The listing builds one solid part. Answer for the finished solid, in the listing's coordinates (mm). A direction names the side the tool comes from. Coordinates: 2 decimals unless noted, no trailing zeros. Loops run counter-clockwise (first coordinate to the right, second up) from the corner with the lowest first, then second, coordinate; pieces in that order, holes last. Notation, with made-up numbers: (68, -23) -> (84, -23) arc R28 ccw to (84, -5) -> close; hole circle Ø2 at (55.5, 70.5). An arc over 180 degrees is marked (long way). Answer in a Markdown table with one row per item.
```python
from build123d import *

# Parameters (mm, degrees)
SKETCH_1_R                   = 14
EXTRUDE_1_DEPTH              = 6
HOLE_WIZARD_M4_3_D           = 4.5
HOLE_WIZARD_M4_3_CBORE_D     = 8
HOLE_WIZARD_M4_3_CBORE_DEPTH = 4.4
PATTERN_CIRCULAR_1_COUNT     = 4
CHAMFER_1_SIZE               = 0.2


with BuildPart() as part:
    # 草圖1 → 填料-伸長1 (new body)
    with BuildSketch(Plane.XY):
        Polygon((-19.2, 16.2), (-16.2, 19.2), (16.2, 19.2), (19.2, 16.2), (19.2, -16.2), (16.2, -19.2), (-16.2, -19.2), (-19.2, -16.2), align=None)
        Circle(SKETCH_1_R, mode=Mode.SUBTRACT)
    extrude(amount=EXTRUDE_1_DEPTH)

    # M4 六角承窩頭蓋螺釘的柱孔3 (through all)
    with Locations(Plane.XY.offset(6)):
        with Locations((-13.435028843, 13.435028843)):
            hole_wizard_m4_3 = CounterBoreHole(HOLE_WIZARD_M4_3_D / 2, HOLE_WIZARD_M4_3_CBORE_D / 2, HOLE_WIZARD_M4_3_CBORE_DEPTH)

    # 環狀複製排列1: M4 六角承窩頭蓋螺釘的柱孔3 ×4 about axis
    pattern_circular_1_axis = Axis((0, 0, 0), (0, 0, 1))
    for i in range(1, PATTERN_CIRCULAR_1_COUNT):
        add(hole_wizard_m4_3.rotate(pattern_circular_1_axis, i * 360 / PATTERN_CIRCULAR_1_COUNT), mode=Mode.SUBTRACT)

    # 導角1
    chamfer_1_edges = [part.edges().sort_by_distance(p)[0] for p in [
        (0, -19.2, 6),
        (17.7, -17.7, 6),
        (19.2, 0, 6),
        (17.7, 17.7, 6),
        (-14, 0, 6),
        (0, 19.2, 6),
        (-17.7, 17.7, 6),
        (-17.435028843, 13.435028843, 6),
        (-13.435028843, -17.435028843, 6),
        (-19.2, 0, 6),
        (17.435028843, -13.435028843, 6),
        (13.435028843, 17.435028843, 6),
        (-17.7, -17.7, 6),
    ]]
    chamfer(chamfer_1_edges, length=CHAMFER_1_SIZE)


solid = part.part
```
Item 1: Find the intervals of material crossed by probe 1 along Y at (x, z) = (0, 3); probe 2 along X at (y, z) = (13, 3.25); probe 3 along Y at (x, z) = (-14.5, 4.25), in increasing order.
Findings below:
| item | result |
|---|---|
| probe 1 | y = -19.2 to -14, 14 to 19.2 |
| probe 2 | x = -19.2 to -17.41, -9.46 to -5.2, 5.2 to 9.46, 17.41 to 19.2 |
| probe 3 | y = -19.2 to -17.29, -9.58 to 9.58, 17.29 to 19.2 |
Item 2: A flat-ended cylindrical pin translates along its axis: pin 1 Ø2.5 at (x, y) = (-13, 12.5) entering from +Z. Find the tip coordinate at first contact, or state that the pin passes through.
Findings below:
| item | result |
|---|---|
| pin 1 | stops at z = 1.6 |
Item 3: A cutting plane is placed at A-A, the plane x = 0. Determine the outline of the cut face in (y, z).
Findings below:
| item | result |
|---|---|
| outline | (-19.2, 0) -> (-14, 0) -> (-14, 5.8) -> (-14.2, 6) -> (-19, 6) -> (-19.2, 5.8) -> close; (14, 0) -> (19.2, 0) -> (19.2, 5.8) -> (19, 6) -> (14.2, 6) -> (14, 5.8) -> close |
Item 4: A cutting plane is placed at D-D, the plane y = -15. Count the separate pieces of the cut face and the enclosed holes in it, plus the area to 3 significant figures.
Findings below:
| item | result |
|---|---|
| separate pieces | 3 |
| enclosed holes | 0 |
| area | 155 mm2 |
Item 5: A cutting plane is placed at C-C, the plane z = 4. Determine the outline of the cut face in (x, y).
Findings below:
| item | result |
|---|---|
| outline | (-19.2, -16.2) -> (-16.2, -19.2) -> (16.2, -19.2) -> (19.2, -16.2) -> (19.2, 16.2) -> (16.2, 19.2) -> (-16.2, 19.2) -> (-19.2, 16.2) -> close; hole circle Ø8 at (-13.44, -13.44); hole circle Ø8 at (-13.44, 13.44); hole circle Ø28 at (0, 0); hole circle Ø8 at (13.44, -13.44); hole circle Ø8 at (13.44, 13.44) |
Item 6: A tool of negligible diameter and unlimited length cuts with its end or side. For faces 4 (the face through (-11.7, 11.7, 1.6)), 5 (the face through (-8, -13, 0)), from which of +Z, -Z, +X, -X, +Y, -Y can it reach the whole face along a straight path? Write none if from no direction.
Findings below:
| item | result |
|---|---|
| face 4 | +Z |
| face 5 | -Z, +X, -X, +Y, -Y |
Item 7: Determine the mould class of faces 1 (the face through (-8, 13, 6)), 2 (the face through (-17.7, -17.7, 2.9)), 3 (the face through (-11.239, -12.947, 0.789)) for opening direction X: +X half, -X half, draft (parallel to the pull), parting line (faces both ways), or undercut.
Findings below:
| item | result |
|---|---|
| face 1 | draft |
| face 2 | -X half |
| face 3 | undercut |
